Here's how the part is built. I have some questions about the finished solid (model axes, mm). Give positions to 0.01 mm unless a question says otherwise; leave off trailing zeros. Write each loop counter-clockwise with the first axis right and the second up, starting at its lowest first coordinate (ties: lowest second). Pieces come first, ordered by that corner, then holes. Notation, with made-up numbers: (87, 89.5) - (120, 89.5) arc R20 cw to (120, 117.5) - close; hole circle Ø9 at (63.5, -24.5). An arc over 180 degrees is marked (long way). Use a Markdown table: item, result.
```python
from build123d import *

# Parameters (mm, degrees)
ESBO_O2_W                = 50
ESBO_O2_H                = 50
RESSALTO_EXTRUS_O2_DEPTH = 10
ESBO_O5_R                = 2.5
CORTE_EXTRUS_O5_DEPTH    = 37.742346142
ESBO_O6_R                = 4
CORTE_EXTRUS_O6_DEPTH    = 10


with BuildPart() as part:
    # Esboço2 → Ressalto-extrusão2 (new body)
    with BuildSketch(Plane(origin=(0, 0, 0), x_dir=(1, 0, 0), z_dir=(0, 1, 0))):
        Rectangle(ESBO_O2_W, ESBO_O2_H)
    extrude(amount=RESSALTO_EXTRUS_O2_DEPTH)

    # Esboço5 → Corte-extrusão5 (cut, through all)
    with BuildSketch(Plane(origin=(0, 10, 0), x_dir=(1, 0, 0), z_dir=(0, 1, 0))):
        with Locations(Location((10, 18.25, 0), (0, 0, 270))):
            Circle(ESBO_O5_R)
        with Locations(Location((10, -18.25, 0), (0, 0, 270))):
            Circle(ESBO_O5_R)
    extrude(amount=-CORTE_EXTRUS_O5_DEPTH, mode=Mode.SUBTRACT)

    # Esboço6 → Corte-extrusão6 (cut)
    with BuildSketch(Plane(origin=(0, 10, 0), x_dir=(1, 0, 0), z_dir=(0, 1, 0))):
        with Locations(Location((10, 0, 0), (0, 0, 270))):
            Circle(ESBO_O6_R)
    extrude(amount=-CORTE_EXTRUS_O6_DEPTH, mode=Mode.SUBTRACT)


solid = part.part
```
Item 1: I need wall thicknesses on line 1 along X through (y, z) = (4, 18.5); line 2 along Z through (x, y) = (11.5, 7.25); line 3 along X through (y, z) = (6, -2). Which ranges of each line are inside material? Lowest first, please. Write a range as [from, to].
Values:
| item | result |
|---|---|
| line 1 | x = [-25, 7.51], [12.49, 25] |
| line 2 | z = [-25, -20.25], [-16.25, -3.71], [3.71, 16.25], [20.25, 25] |
| line 3 | x = [-25, 6.54], [13.46, 25] |
Item 2: If we section it at B-B, the plane y = 5.75: Write out the boundary of the cut face in (x, z).
Values:
| item | result |
|---|---|
| outline | (-25, -25) - (25, -25) - (25, 25) - (-25, 25) - close; hole circle Ø8 at (10, 0); hole circle Ø5 at (10, -18.25); hole circle Ø5 at (10, 18.25) |
Item 3: Thinking about a two-plate mould opening in X: for faces 1 (the flat face through (25, 5, 0)), 2 (the cylindrical face through (8.479, 5.07, -20.234)), 3 (the flat face through (0, 5, 25)), which applies, +X half, -X half, draft (parallel to the pull), parting line (faces both ways), or undercut?
Values:
| item | result |
|---|---|
| face 1 | +X half |
| face 2 | undercut |
| face 3 | draft |
Item 4: If we section it at C-C, the plane x = 10: Write out the boundary of the cut face in (y, z).
Values:
| item | result |
|---|---|
| outline | (0, -25) - (10, -25) - (10, -20.75) - (0, -20.75) - close; (0, -15.75) - (10, -15.75) - (10, -4) - (0, -4) - close; (0, 4) - (10, 4) - (10, 15.75) - (0, 15.75) - close; (0, 20.75) - (10, 20.75) - (10, 25) - (0, 25) - close |
Item 5: If we section it at D-D, the plane z = -18.25: Write out the boundary of the cut face in (x, y), plus the area to 3 significant figures.
Values:
| item | result |
|---|---|
| outline | (-25, 0) - (7.5, 0) - (7.5, 10) - (-25, 10) - close; (12.5, 0) - (25, 0) - (25, 10) - (12.5, 10) - close |
| area | 450 mm2 |
Item 6: If we section it at A-A, the plane z = 0: Write out the boundary of the cut face in (x, y).
Values:
| item | result |
|---|---|
| outline | (-25, 0) - (6, 0) - (6, 10) - (-25, 10) - close; (14, 0) - (25, 0) - (25, 10) - (14, 10) - close |
